Read the model definition and answer for the solid it produces. Units are mm, in the model's axes. A direction names the side the tool comes from. Coordinates: 2 decimals unless noted, no trailing zeros. Write each loop counter-clockwise with the first axis right and the second up, starting at its lowest first coordinate (ties: lowest second). Pieces come first, ordered by that corner, then holes.
(1) Section B-B on y = 1.95 is taken. Write down the section's boundary in (x, z), then the cut area to 3 significant figures.
(2) Find the intervals of material crossed by probe 1 along X at (y, z) = (1.8, -1.75); probe 2 along Y at (x, z) = (-8.5, -6.25); probe 3 along X at (y, z) = (0.8, 0), in increasing order.
(3) Which of the six approach directions +Z, -Z, +X, -X, +Y, -Y give full straight-line access (tool end or side, diameter ignored) to faces 4 (the flat face through (8, 2, 0.5)), 5 (the flat face through (-18, 2, -6.5)), 6 (the flat face through (13, 2, -8.5)), 7 (the flat face through (46, 2, -6.5))?
(4) The mould has two halves that part along X. Classify faces 1 (the flat face through (65, 2, -7)), 2 (the flat face through (15, 2, -6.5)), 3 (the flat face through (14, 4, -7)): +X half, -X half, draft (parallel to the pull), parting line (faces both ways), or undercut.
(5) Section A-A on x = 39.5 is taken. Write down the section's boundary in (y, z).
(6) Given pin 1 (0.9 mm diameter, centred on x = -25.5, y = 3, fed in from +Z); pin 2 (0.9 mm diameter, centred on y = 3, z = -3, fed in from -X); pin 3 (1.5 mm diameter, centred on y = 2, z = -1.5, fed in from +X), each flat-ended and moving along its own axis, determine where each tip first touches the part or whether it passes through.
(7) Section C-C on x = 12 is taken. Write down the section's boundary in (y, z), then the cut area to 3 significant figures.
from build123d import *

# Parameters (mm, degrees)
SKETCH_1_R          = 1.6
EXTRUDE_1_DEPTH     = 1
SKETCH_2_W          = 102
SKETCH_2_H          = 2
EXTRUDE_2_DEPTH     = 3
SKETCH_3_W          = 2
SKETCH_3_H          = 7
EXTRUDE_3_DEPTH     = 3
FILLET_1_R          = 5
FILLET_2_R          = 2
CUT_EXTRUDE_1_REACH = 67.833


with BuildPart() as part:
    # 草图1 → 凸台-拉伸1 (new body)
    with BuildSketch(Plane(origin=(0, 0, 0), x_dir=(1, 0, 0), z_dir=(0, 1, 0))):
        Polygon((-37, 10), (-37, 5), (-5, 5), (-5, -3), (35, -3), (35, 5), (65, 5), (65, 10), align=None)
        with Locations(Location((0, 0, 0), (0, 0, 270))):
            Circle(SKETCH_1_R, mode=Mode.SUBTRACT)
        with Locations(Location((30, 0, 0), (0, 0, 270))):
            Circle(SKETCH_1_R, mode=Mode.SUBTRACT)
    extrude(amount=EXTRUDE_1_DEPTH)

    # 草图2 → 凸台-拉伸2 (add)
    with BuildSketch(Plane(origin=(0, 1, 0), x_dir=(1, 0, 0), z_dir=(0, 1, 0))):
        with Locations((14, 7.5)):
            Rectangle(SKETCH_2_W, SKETCH_2_H)
    extrude(amount=EXTRUDE_2_DEPTH)

    # 草图3 → 凸台-拉伸3 (add)
    with BuildSketch(Plane(origin=(0, 1, 0), x_dir=(1, 0, 0), z_dir=(0, 1, 0))):
        with Locations((8, 3)):
            Rectangle(SKETCH_3_W, SKETCH_3_H)
        with Locations((22, 3)):
            Rectangle(SKETCH_3_W, SKETCH_3_H)
    extrude(amount=EXTRUDE_3_DEPTH)

    # 圆角1
    fillet_1_edges = [part.edges().sort_by_distance(p)[0] for p in [
        (35, 0.5, 3),
        (-5, 0.5, 3),
        (7, 2.5, -6.5),
        (23, 2.5, -6.5),
    ]]
    fillet(fillet_1_edges, radius=FILLET_1_R)

    # 圆角2
    fillet_2_edges = [part.edges().sort_by_distance(p)[0] for p in [
        (9, 2.5, -6.5),
        (21, 2.5, -6.5),
    ]]
    fillet(fillet_2_edges, radius=FILLET_2_R)

    # 草图4 → 切除-拉伸1 (cut, up to next)
    with BuildSketch(Plane(origin=(0, 1, 0), x_dir=(1, 0, 0), z_dir=(0, 1, 0)), mode=Mode.PRIVATE) as cut_extrude_1_sk1:
        with BuildLine():
            Line((23, -3), (30, -3))
            ThreePointArc((30, -3), (33.535533906, -1.535533906), (35, 2))
            Line((35, 2), (35, 5))
            Line((35, 5), (24.429285786, 5))
            ThreePointArc((24.429285786, 5), (23.371092404, 3.390294809), (23, 1.5))
            Line((23, 1.5), (23, -0.5))
            Line((23, -0.5), (23, -3))
        make_face()
    cut_extrude_1_tool1 = extrude(cut_extrude_1_sk1.sketch, amount=-CUT_EXTRUDE_1_REACH, mode=Mode.PRIVATE) & part.part
    add(cut_extrude_1_tool1.solids().sort_by_distance((28.803609, 1, -1.118494))[0], mode=Mode.SUBTRACT)


solid = part.part
Response:
1. outline: (-37, -8.5) - (65, -8.5) - (65, -6.5) - (28, -6.5) arc R5 cw to (23, -1.5) - (23, 0.5) - (21, 0.5) - (21, -4.5) arc R2 cw to (19, -6.5) - (11, -6.5) arc R2 cw to (9, -4.5) - (9, 0.5) - (7, 0.5) - (7, -1.5) arc R5 cw to (2, -6.5) - (-37, -6.5) - close
1. area: 244 mm2
2. probe 1: x = 6.99 to 9, 21 to 23.01
2. probe 2: y = 0 to 1
2. probe 3: x = -4.58 to -1.6, 1.6 to 23
3. face 4: +Z, +X, -X, +Y
3. face 5: +Z, -X, +Y
3. face 6: -Z, +X, -X, +Y
3. face 7: +Z, +X, +Y
4. face 1: +X half
4. face 2: undercut
4. face 3: draft
5. outline: (0, -10) - (1, -10) - (1, -8.5) - (4, -8.5) - (4, -6.5) - (1, -6.5) - (1, -5) - (0, -5) - close
6. pin 1: stops at z = -6.5
6. pin 2: stops at x = 6.6
6. pin 3: stops at x = 23.06
7. outline: (0, -10) - (1, -10) - (1, -8.5) - (4, -8.5) - (4, -6.5) - (1, -6.5) - (1, 3) - (0, 3) - close
7. area: 19.0 mm2
